from build123d import *

# Parameters (mm, degrees)
SKETCH1_W           = 45
SKETCH1_H           = 40
BOSS_EXTRUDE1_DEPTH = 5
CHAMFER1_SIZE       = 5
CHAMFER1_SIZE_2     = 18.660254038
SKETCH2_W           = 45
SKETCH2_H           = 3
BOSS_EXTRUDE2_DEPTH = 7
FILLET1_R           = 3


with BuildPart() as part:
    # Sketch1 → Boss-Extrude1 (new body)
    with BuildSketch(Plane(origin=(0, 0, 0), x_dir=(1, 0, 0), z_dir=(0, 1, 0))):
        Rectangle(SKETCH1_W, SKETCH1_H)
    extrude(amount=BOSS_EXTRUDE1_DEPTH)

    # Chamfer1
    # the kernel refuses this chamfer: 18.660254038, 5 mm, written as the material it takes off along each edge
    with BuildSketch(Plane(origin=(-70.955484165, 5, -20), x_dir=(0, -0.9905000388259539, -0.13751244702129164), z_dir=(1, 0, 0))) as chamfer1_piece_1:
        Polygon((CHAMFER1_SIZE * 0.990500038826, -CHAMFER1_SIZE * 0.137512447021), (-CHAMFER1_SIZE_2 * 0.13751244702, -CHAMFER1_SIZE_2 * 0.990500038818), (0, 0), align=None)
    extrude(amount=141.910968331, mode=Mode.SUBTRACT)

    # Sketch2 → Boss-Extrude2 (add)
    with BuildSketch(Plane(origin=(0, 5, 0), x_dir=(1, 0, 0), z_dir=(0, 1, 0))):
        with Locations((0, -18.5)):
            Rectangle(SKETCH2_W, SKETCH2_H)
    extrude(amount=BOSS_EXTRUDE2_DEPTH)

    # Fillet1
    fillet1_edges = [part.edges().sort_by_distance(p)[0] for p in [
        (0, 5, 17),
    ]]
    fillet(fillet1_edges, radius=FILLET1_R)


solid = part.part
CAD build for the part. Positions are in the model's coordinates, mm. A direction names the side the tool comes from. Give positions to 0.01 mm unless a question says otherwise; leave off trailing zeros. Order: outer loops, then holes, each group sorted by start corner. A loop starts at its lowest first (then second) coordinate and runs counter-clockwise, first axis right, second up. Notation, with made-up numbers: (70, 50) -> (79, 50) arc R17 ccw to (79, 55) -> close; hole circle Ø6 at (63, 54.5). An arc over 180 degrees is marked (long way). Return JSON: item names as keys, results as strings.
Q1. Saw through at A-A (x = 11). Write the cut outline in (y, z).
Working result:
{"outline": "(0, -20) -> (5, -1.34) -> (5, 14) arc R3 cw to (8, 17) -> (12, 17) -> (12, 20) -> (0, 20) -> close"}
Q2. Drill centre lines: line 1 (Y direction, x = 20, z = 13); line 2 (Z direction, x = -2, y = 11.75); line 3 (Z direction, x = 11.5, y = 6.25). Where is each one in solid material? Low to high.
Working result:
{"line 1": "0 to 5", "line 2": "17 to 20", "line 3": "16.44 to 20"}
Q3. Saw through at C-C (z = 11). Write the cut outline in (x, y), then the cut area to 3 significant figures.
Working result:
{"outline": "(-22.5, 0) -> (22.5, 0) -> (22.5, 5) -> (-22.5, 5) -> close", "area": "225 mm²"}
Q4. Flat gauge pins, fed straight in: pin 1 (4 mm diameter, centred on x = 8.5, z = -4, fed in from +Y); pin 2 (2 mm diameter, centred on x = -5, y = 9.5, fed in from -Z); pin 3 (1.5 mm diameter, centred on x = 13.5, z = -8.5, fed in from +Y). Where does each tip first touch, or does it go through?
Working result:
{"pin 1": "y = 4.82", "pin 2": "z = 17", "pin 3": "y = 3.28"}
Q5. Saw through at B-B (y = 8.75). Write the cut outline in (x, z), then the cut area to 3 significant figures.
Working result:
{"outline": "(-22.5, 17) -> (22.5, 17) -> (22.5, 20) -> (-22.5, 20) -> close", "area": "135 mm²"}
Q6. Which spindle directions (+Z, -Z, +X, -X, +Y, -Y) get a long thin tool onto all of the face, cutting with end or side? Do faces 1 (the face through (22.5, 3, 5)), 2 (the face through (0, 10, 17)). Say none if no direction does.
Working result:
{"face 1": "+Z, -Z, +X, +Y, -Y", "face 2": "-Z, +X, -X, +Y"}
